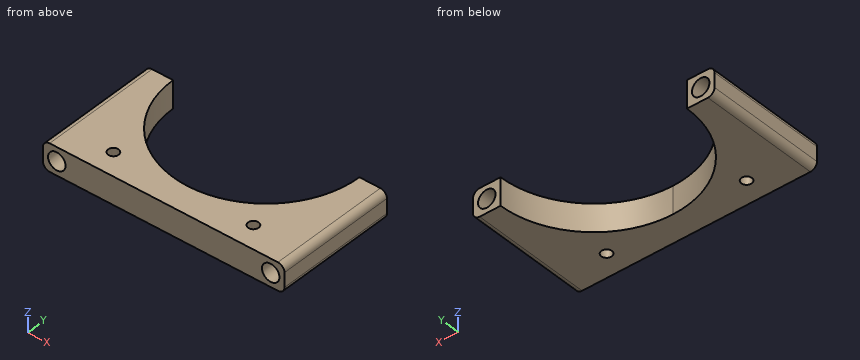
from build123d import *

# Parameters (mm, degrees)
BOSS_EXTRUDE1_DEPTH = 25
SKETCH5_R           = 7.94
CUT_EXTRUDE1_DEPTH  = 5000
SKETCH6_R           = 4.7625
CUT_EXTRUDE2_DEPTH  = 5000
FILLET2_R           = 6


with BuildPart() as part:
    # Sketch4 → Boss-Extrude1 (new body)
    with BuildSketch(Plane.XY):
        with BuildLine():
            ThreePointArc((0, -25), (-77.42819254, 7.07180746), (-109.5, 84.5))
            Line((-109.5, 84.5), (-109.5, -25))
            Line((-109.5, -25), (0, -25))
        make_face()
        with BuildLine():
            ThreePointArc((84.5, 84.5), (59.75052301, 24.74947699), (0, 0))
            ThreePointArc((0, 0), (-59.75052301, 24.74947699), (-84.5, 84.5))
            Line((-84.5, 84.5), (-109.5, 84.5))
            ThreePointArc((-109.5, 84.5), (-77.42819254, 7.07180746), (0, -25))
            ThreePointArc((0, -25), (77.42819254, 7.07180746), (109.5, 84.5))
            Line((109.5, 84.5), (84.5, 84.5))
        make_face()
        with BuildLine():
            Line((109.5, -25), (109.5, 84.5))
            ThreePointArc((109.5, 84.5), (77.42819254, 7.07180746), (0, -25))
            Line((0, -25), (109.5, -25))
        make_face()
    extrude(amount=BOSS_EXTRUDE1_DEPTH)

    # Sketch5 → Cut-Extrude1 (cut)
    with BuildSketch(Plane(origin=(0, 84.5, 0), x_dir=(1, 0, 0), z_dir=(0, 1, 0))):
        with Locations((-97, -12.5)):
            Circle(SKETCH5_R)
        with Locations((97, -12.5)):
            Circle(SKETCH5_R)
    extrude(amount=-CUT_EXTRUDE1_DEPTH, mode=Mode.SUBTRACT)

    # Sketch6 → Cut-Extrude2 (cut)
    with BuildSketch(Plane.XY.offset(25)):
        with Locations((-63.5, -4)):
            Circle(SKETCH6_R)
        with Locations((63.5, -4)):
            Circle(SKETCH6_R)
    extrude(amount=-CUT_EXTRUDE2_DEPTH, mode=Mode.SUBTRACT)

    # Fillet2
    fillet2_edges = [part.edges().sort_by_distance(p)[0] for p in [
        (109.5, 29.75, 25),
        (-109.5, 29.75, 25),
        (-109.5, 29.75, 0),
        (109.5, 29.75, 0),
    ]]
    fillet(fillet2_edges, radius=FILLET2_R)


solid = part.part
The model under review builds one solid part; all positions refer to its coordinate system, in mm. Coordinates: 2 decimals unless noted, no trailing zeros. Write each loop counter-clockwise with the first axis right and the second up, starting at its lowest first coordinate (ties: lowest second). Pieces come first, ordered by that corner, then holes. Notation, with made-up numbers: (-27.75, 89.5) - (15.25, 89.5) arc R13 ccw to (15.25, 101.5) - close; hole circle Ø11 at (84.25, -20). An arc over 180 degrees is marked (long way). Answer as a JSON object with one key per item and string values. Group by question number.
1. To check wall thickness, follow probe 1 along X at (y, z) = (-14, 19); probe 2 along X at (y, z) = (76, 13.75); probe 3 along X at (y, z) = (54.5, 12). State the ranges of each line that lie inside material, in increasing order.
2. Add section B-B (x = 97). Give the boundary of the cut face in (y, z), plus the area to 3 significant figures.
3. Add section A-A (y = -4). Give the boundary of the cut face in (x, z).
4. Clearance check with a flat-ended pin moving along its axis: pin 1 Ø10 at (x, z) = (-27, 5) entering from +Y. State where the tip first meets the part, or that it passes through.
5. Add section C-C (z = 12.5). Give the boundary of the cut face in (x, y) (1 decimal).
6. Add section D-D (y = 18). Give the boundary of the cut face in (x, z).
Findings:
{
 "1": {"probe 1": "-109.5 to -101.56, -92.44 to 92.44, 101.56 to 109.5", "probe 2": "-109.5 to -104.84, -89.16 to -84.07, 84.07 to 89.16, 104.84 to 109.5", "probe 3": "-109.5 to -104.92, -89.08 to -79, 79 to 89.08, 104.92 to 109.5"},
 "2": {"outline": "(-25, 0) - (84.5, 0) - (84.5, 4.56) - (-25, 4.56) - close; (-25, 20.44) - (84.5, 20.44) - (84.5, 25) - (-25, 25) - close", "area": "999 mm²"},
 "3": {"outline": "(-109.5, 6) arc R6 ccw to (-103.5, 0) - (-68.26, 0) - (-68.26, 25) - (-103.5, 25) arc R6 ccw to (-109.5, 19) - close; (-58.74, 0) - (58.74, 0) - (58.74, 25) - (-58.74, 25) - close; (68.26, 0) - (103.5, 0) arc R6 ccw to (109.5, 6) - (109.5, 19) arc R6 ccw to (103.5, 25) - (68.26, 25) - close; hole circle Ø15.88 at (-97, 12.5); hole circle Ø15.88 at (97, 12.5)"},
 "4": {"pin 1": "y = 6.29"},
 "5": {"outline": "(-109.5, -25) - (-104.9, -25) - (-104.9, 84.5) - (-109.5, 84.5) - close; (-89.1, -25) - (89.1, -25) - (89.1, 84.5) - (84.5, 84.5) arc R84.5 cw to (-84.5, 84.5) - (-89.1, 84.5) - close; (104.9, -25) - (109.5, -25) - (109.5, 84.5) - (104.9, 84.5) - close; hole circle Ø9.5 at (-63.5, -4); hole circle Ø9.5 at (63.5, -4)"},
 "6": {"outline": "(-109.5, 6) arc R6 ccw to (-103.5, 0) - (-52.13, 0) - (-52.13, 25) - (-103.5, 25) arc R6 ccw to (-109.5, 19) - close; (52.13, 0) - (103.5, 0) arc R6 ccw to (109.5, 6) - (109.5, 19) arc R6 ccw to (103.5, 25) - (52.13, 25) - close; hole circle Ø15.88 at (-97, 12.5); hole circle Ø15.88 at (97, 12.5)"}
}
